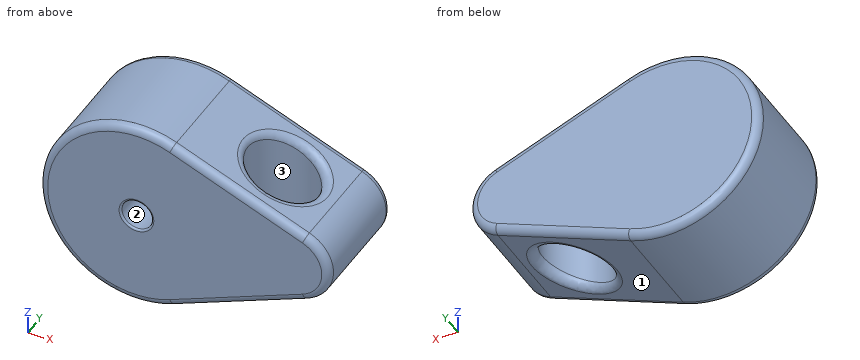
from build123d import *

# Parameters (mm, degrees)
SKETCH1_R               = 1.016
BOSS_EXTRUDE1_DEPTH     = 7.62
SKETCH2_R               = 1.016
BOSS_EXTRUDE2_DEPTH     = 1.5875
SKETCH3_R               = 2.286
CUT_EXTRUDE1_DEPTH      = 7.35
CUT_EXTRUDE1_DEPTH_BACK = 7.35
FILLET1_R               = 0.508
FILLET2_R               = 0.127


with BuildPart() as part:
    # Sketch1 → Boss-Extrude1 (new body)
    with BuildSketch(Plane(origin=(0, 0, 0), x_dir=(1, 0, 0), z_dir=(0, 1, 0))):
        with BuildLine():
            Line((11.1125, 2.35464302), (2.38125, 5.886607549))
            ThreePointArc((2.38125, 5.886607549), (-6.35, 0), (2.38125, -5.886607549))
            Line((2.38125, -5.886607549), (11.1125, -2.35464302))
            ThreePointArc((11.1125, -2.35464302), (12.7, 0), (11.1125, 2.35464302))
        make_face()
        Circle(SKETCH1_R, mode=Mode.SUBTRACT)
    extrude(amount=BOSS_EXTRUDE1_DEPTH)

    # Sketch2 → Boss-Extrude2 (add)
    with BuildSketch(Plane(origin=(0, 7.62, 0), x_dir=(1, 0, 0), z_dir=(0, 1, 0))):
        Circle(SKETCH2_R)
    extrude(amount=-BOSS_EXTRUDE2_DEPTH)

    # Sketch3 → Cut-Extrude1 (cut, two sides)
    with BuildSketch(Plane.XY) as cut_extrude1_sk:
        with Locations((7.62, 3.81)):
            Circle(SKETCH3_R)
    extrude(amount=CUT_EXTRUDE1_DEPTH, mode=Mode.SUBTRACT)
    extrude(cut_extrude1_sk.sketch, amount=-CUT_EXTRUDE1_DEPTH_BACK, mode=Mode.SUBTRACT)

    # Fillet1
    fillet1_edges = [part.edges().sort_by_distance(p)[0] for p in [
        (6.746875, 0, -4.120625284),
        (6.746875, 7.62, -4.120625284),
        (5.334, 3.809986249, -4.692161363),
        (5.334, 3.810013751, 4.692161363),
        (6.746875, 0, 4.120625284),
        (6.746875, 7.62, 4.120625284),
        (-6.35, 0, 0),
        (-6.35, 7.62, 0),
        (12.7, 7.62, 0),
        (12.7, 0, 0),
    ]]
    fillet(fillet1_edges, radius=FILLET1_R)

    # Fillet2
    fillet2_edges = [part.edges().sort_by_distance(p)[0] for p in [
        (-1.016, 0, 0),
    ]]
    fillet(fillet2_edges, radius=FILLET2_R)


solid = part.part
Design review of the part built by this model. Coordinates are the model's own, in mm. Face numbers are marked on the shaded views. Give positions to 0.01 mm unless a question says otherwise; leave off trailing zeros. Order: outer loops, then holes, each group sorted by start corner. A loop starts at its lowest first (then second) coordinate and runs counter-clockwise, first axis right, second up.
1. To check wall thickness, follow L1, parallel to Z at x = 0, y = 2.15; L2, parallel to Y at x = 7.62, z = 1; L3, parallel to X at y = 3.81, z = -1.75. State the ranges of each line that lie inside material, in increasing order.
Solution:
L1: z = -6.35 to -1.02, 1.02 to 6.35
L2: y = 0 to 1.52, 6.1 to 7.62
L3: x = -6.1 to 5.33, 9.91 to 12
2. Add section B-B, the plane y = 3.81. State how many separate pieces and enclosed holes the cut face has, then the cut area to 3 significant figures.
Solution:
separate pieces: 2
enclosed holes: 1
area: 132 mm2
3. For pin 1 Ø2.5 at (x, z) = (0, 0) entering from -Y; pin 2 Ø1.5 at (y, z) = (6, -1.5) entering from -X; pin 3 Ø1 at (y, z) = (4, 3.5) entering from -X, all flat-tipped, find the tip position at first contact; note any pin that passes through.
Solution:
pin 1: stops at y = 0
pin 2: stops at x = -6.31
pin 3: stops at x = -5.6
4. Mouldability with a two-part tool opening along Z and no side actions: class the marked faces 1, 2 and 3 as +Z half, -Z half, draft (parallel to the pull), parting line (faces both ways), or undercut.
Solution:
face 1: -Z half
face 2: undercut
face 3: draft
5. Add section A-A, the plane z = 0. State the section outline as (x, y) points.
Solution:
outline: (-6.35, 0.51) arc R0.51 ccw to (-5.84, 0) - (-1.14, 0) arc R0.13 ccw to (-1.02, 0.13) - (-1.02, 6.03) - (1.02, 6.03) - (1.02, 0.13) arc R0.13 ccw to (1.14, 0) - (12.19, 0) arc R0.51 ccw to (12.7, 0.51) - (12.7, 7.11) arc R0.51 ccw to (12.19, 7.62) - (-5.84, 7.62) arc R0.51 ccw to (-6.35, 7.11) - close; hole circle Ø4.57 at (7.62, 3.81)
